Read the model definition and answer for the solid it produces. Units are mm, in the model's axes. A direction names the side the tool comes from. Coordinates: 2 decimals unless noted, no trailing zeros. Loops run counter-clockwise (first coordinate to the right, second up) from the corner with the lowest first, then second, coordinate; pieces in that order, holes last. Notation, with made-up numbers: M -32.75,80.25 L -10.75,80.25 A15 cw -10.75,87.25 Z; hole C 56,35 d2. An arc over 180 degrees is marked long. Put each result on its own line as item: value.
from build123d import *

# Parameters (mm, degrees)
SKETCH1_R           = 18.5
BOSS_EXTRUDE1_DEPTH = 12
SKETCH2_R           = 6
CUT_EXTRUDE1_DEPTH  = 12
SKETCH3_R           = 15
SKETCH3_R_2         = 9.5
CUT_EXTRUDE2_DEPTH  = 1
CUT_EXTRUDE3_START  = -1
SKETCH4_R           = 15
SKETCH4_R_2         = 9.5
CUT_EXTRUDE3_DEPTH  = 1


with BuildPart() as part:
    # Sketch1 → Boss-Extrude1 (new body)
    with BuildSketch(Plane.XY):
        Circle(SKETCH1_R)
    extrude(amount=BOSS_EXTRUDE1_DEPTH)

    # Sketch2 → Cut-Extrude1 (cut)
    with BuildSketch(Plane.XY.offset(12)):
        Circle(SKETCH2_R)
    extrude(amount=-CUT_EXTRUDE1_DEPTH, mode=Mode.SUBTRACT)

    # Sketch3 → Cut-Extrude2 (cut)
    with BuildSketch(Plane.XY.offset(12)):
        Circle(SKETCH3_R)
        Circle(SKETCH3_R_2, mode=Mode.SUBTRACT)
    extrude(amount=-CUT_EXTRUDE2_DEPTH, mode=Mode.SUBTRACT)

    # Sketch4 → Cut-Extrude3 (cut)
    with BuildSketch(Plane(origin=(0, 0, 0), x_dir=(-1, 0, 0), z_dir=(0, 0, -1)).offset(CUT_EXTRUDE3_START)):
        with Locations(Location((0, 0, 0), (0, 0, 180))):
            Circle(SKETCH4_R)
        with Locations(Location((0, 0, 0), (0, 0, 180))):
            Circle(SKETCH4_R_2, mode=Mode.SUBTRACT)
    extrude(amount=CUT_EXTRUDE3_DEPTH, mode=Mode.SUBTRACT)


solid = part.part
1) Given pin 1 Ø2 at (y, z) = (-0.5, 8.5) entering from +X; pin 2 Ø4 at (x, z) = (9, 3) entering from +Y; pin 3 Ø2 at (y, z) = (8.5, 6) entering from +X; pin 4 Ø4 at (x, y) = (10, -6) entering from +Z, each flat-ended and moving along its own axis, determine where each tip first touches the part or whether it passes through.
Answer list:
pin 1: stops at x = 18.5
pin 2: stops at y = 17.12
pin 3: stops at x = 16.91
pin 4: stops at z = 11
2) Find section D-D, the plane y = 11. Write down the section's boundary in (x, z), plus the area to 3 significant figures.
Answer list:
outline: M -14.87,0 L -10.2,0 L -10.2,1 L 10.2,1 L 10.2,0 L 14.87,0 L 14.87,12 L 10.2,12 L 10.2,11 L -10.2,11 L -10.2,12 L -14.87,12 Z
area: 316 mm^2
3) Which of the six approach directions +Z, -Z, +X, -X, +Y, -Y give full straight-line access (tool end or side, diameter ignored) to faces 1 (the cylindrical face through (8.06, -12.65, 0.51)), 2 (the cylindrical face through (-14.985, 0.66, 11.507)), 3 (the cylindrical face through (-6, 0, 6))?
Answer list:
face 1: -Z
face 2: +Z
face 3: +Z, -Z
4) Find section A-A, the plane y = 0. Write down the section's boundary in (x, z), plus the area to 3 significant figures.
Answer list:
outline: M -18.5,0 L -15,0 L -15,1 L -9.5,1 L -9.5,0 L -6,0 L -6,12 L -9.5,12 L -9.5,11 L -15,11 L -15,12 L -18.5,12 Z; M 6,0 L 9.5,0 L 9.5,1 L 15,1 L 15,0 L 18.5,0 L 18.5,12 L 15,12 L 15,11 L 9.5,11 L 9.5,12 L 6,12 Z
area: 278 mm^2
5) Determine the mould class of faces 4 (the flat face through (-0.1, -6.2, 0)), 5 (the flat face through (0, 10, 1)), 6 (the cylindrical face through (-4.01, -18.06, 5.92)) for opening direction Y: released by +Y, released by -Y, zero draft, split by the parting line, or undercut.
Answer list:
face 4: zero draft
face 5: undercut
face 6: split by the parting line
6) Find section C-C, the plane z = 2.75. Write down the section's boundary in (x, y), plus the area to 3 significant figures.
Answer list:
outline: C 0,0 d37; hole C 0,0 d12
area: 962 mm^2
7) Straight lines are drawn through the part: line 1 (Y direction, x = 0, z = 0.6); line 2 (Y direction, x = 0, z = 4.5); line 3 (Z direction, x = 9.5, y = -5.5). For each, find the intervals that lie inside material, in ascending order. Write a range as [from, to].
Answer list:
line 1: y = [-18.5, -15], [-9.5, -6], [6, 9.5], [15, 18.5]
line 2: y = [-18.5, -6], [6, 18.5]
line 3: z = [1, 11]
